from build123d import *

# Parameters (mm, degrees)
F0_W     = 35
F0_H     = 35
F1_DEPTH = 5
F2_R     = 3.1
F3_DEPTH = 5.001
F4_W     = 19
F4_H     = 19
F5_DEPTH = 20
F7_DEPTH = 35


with BuildPart() as f1:
    # F0 (on Front) → F1 (new body)
    with BuildSketch(Plane.XZ):
        with Locations((0.559466, -17.5)):
            Rectangle(F0_W, F0_H)
    extrude(amount=F1_DEPTH)

    # F2 (on face) → F3 (cut, through all)
    with BuildSketch(Plane(origin=(0, 0, 0), x_dir=(-1, 0, 0), z_dir=(0, 1, 0))):
        with Locations((-13.059466, -5)):
            Circle(F2_R)
        with Locations((11.940534, -5)):
            Circle(F2_R)
        with Locations((-13.059466, -30)):
            Circle(F2_R)
        with Locations((11.940534, -30)):
            Circle(F2_R)
    extrude(amount=-F3_DEPTH, mode=Mode.SUBTRACT)

    # F4 (on face) → F5 (join)
    with BuildSketch(Plane(origin=(0, 0, 0), x_dir=(-1, 0, 0), z_dir=(0, 1, 0))):
        with Locations((-0.559466, -17.5)):
            Rectangle(F4_W, F4_H)
    extrude(amount=F5_DEPTH)

    # F6 (on face) → F7 (cut)
    with BuildSketch(Plane.YZ.offset(10.059466)):
        Polygon((20, -18.355448), (20, -17.5), (8.076428, -16.147804), (8.076428, -17.003253), align=None)
    extrude(amount=-F7_DEPTH, mode=Mode.SUBTRACT)


solid = f1.part
Here's how the part is built. I have some questions about the finished solid (model axes, mm). A direction names the side the tool comes from. Round coordinates to 2 decimals unless told otherwise and drop trailing zeros. Loops run counter-clockwise (first coordinate to the right, second up) from the corner with the lowest first, then second, coordinate; pieces in that order, holes last. Notation, with made-up numbers: M 14,18.25 L 67,18.25 A37 ccw 67,56.25 Z; hole C 17,84 d9. An arc over 180 degrees is marked long. Write each question's results on one line, items separated by ' | '. Start each with the question number.
(1) On a 3-axis mill with a long thin cutter (end or side, diameter ignored), from which of +Z, -Z, +X, -X, +Y, -Y can I reach the whole of each face in a straight line? I mean faces 5 (the flat face through (-8.941, 10, -18)), 6 (the flat face through (0.7, 8.076, -16.6)), 7 (the flat face through (1, 10, -27)). Say none if no direction works.
(2) I want a section at C-C (x = 0.5). Please give me the cut outline in (y, z), then the cut area to 3 significant figures.
(3) I want a section at B-B (y = -3.5). Please give me the cut outline in (x, z).
(4) Thinking about a two-plate mould opening in Y: for faces 1 (the flat face through (1, 10, -8)), 2 (the flat face through (0.692, 14.122, -16.833)), 3 (the flat face through (0.69, 13.95, -17.67)), 4 (the flat face through (1, 20, -13)), which applies, pulls with the +Y half, pulls with the -Y half, needs draft (parallel to the pull), parting line crosses it, or undercut?
(5) I want a section at A-A (z = -5). Please give me the cut outline in (x, y), then the cut area to 3 significant figures.
(6) Will these pins go through, and if not, where does the flat tip stop? P1, Ø9.5, axis at y = 6, z = -18, coming from the -X side; P2, Ø8, axis at x = -5, y = 7.5, coming from the -Z side; P3, Ø9.5, axis at y = 9, z = -16.5, coming from the +X side; P4, Ø2, axis at y = 1.5, z = -4, coming from the -X side.
(7) I want a section at D-D (y = 16). Please give me the cut outline in (x, z), then the cut area to 3 significant figures.
(8) If I drill on probe 1 along Y at (x, z) = (-10, -10); probe 2 along X at (y, z) = (9.5, -9); probe 3 along Z at (x, y) = (0, 6), over which ranges is the centre line in solid material (lowest first)? Write a range as from..to.
Solved:
1) face 5: +Z, -Z, -X, +Y | face 6: +X, -X | face 7: -Z, +X, -X, +Y
2) outline: M -5,-35 L 0,-35 L 0,-27 L 20,-27 L 20,-18.36 L 8.08,-17 L 8.08,-16.15 L 20,-17.5 L 20,-8 L 0,-8 L 0,0 L -5,0 Z | area: 545 mm²
3) outline: M -16.94,-35 L 18.06,-35 L 18.06,0 L -16.94,0 Z; hole C -11.94,-30 d6.2; hole C -11.94,-5 d6.2; hole C 13.06,-30 d6.2; hole C 13.06,-5 d6.2
4) face 1: needs draft | face 2: undercut | face 3: undercut | face 4: pulls with the +Y half
5) outline: M -16.94,-5 L -15.04,-5 L -15.04,0 L -16.94,0 Z; M -8.84,-5 L 9.96,-5 L 9.96,0 L -8.84,0 Z; M 16.16,-5 L 18.06,-5 L 18.06,0 L 16.16,0 Z | area: 113 mm²
6) P1: stops at x = -8.94 | P2: stops at z = -27 | P3: stops at x = 10.06 | P4: passes through
7) outline: M -8.94,-27 L 10.06,-27 L 10.06,-17.9 L -8.94,-17.9 Z; M -8.94,-17.05 L 10.06,-17.05 L 10.06,-8 L -8.94,-8 Z | area: 345 mm²
8) probe 1: y = -5..0 | probe 2: x = -8.94..10.06 | probe 3: z = -27..-8
